from build123d import *

# Parameters (mm, degrees)
ESBO_O1_W                     = 46
ESBO_O1_H                     = 19
RESSALTO_EXTRUS_O1_DEPTH      = 1.5
CORTE_EXTRUS_O3_DEPTH         = 25.929901725
CORTE_EXTRUS_O3_DEPTH_BACK    = 25.929901725
ESBO_O6_W                     = 3
ESBO_O6_H                     = 6
CORTE_EXTRUS_O2_DEPTH         = 25.929901725
CORTE_EXTRUS_O2_DEPTH_BACK    = 25.929901725
DENTE_W                       = 3
DENTE_H                       = 3
RESSALTO_EXTRUS_O3_DEPTH      = 1.5
RESSALTO_EXTRUS_O3_DEPTH_BACK = 1.5
ESBO_O4_W                     = 3
ESBO_O4_H                     = 6
ESBO_O21_W                    = 9
ESBO_O21_H                    = 3
ESBO_O21_W_2                  = 2.5
ESBO_O21_H_2                  = 5.5
CORTE_EXTRUS_O11_DEPTH        = 3
ESBO_O3_W                     = 3
ESBO_O3_H                     = 4.5
RESSALTO_EXTRUS_O2_DEPTH      = 1.5
CORTE_EXTRUS_O12_DEPTH        = 28.721832551
CORTE_EXTRUS_O12_DEPTH_BACK   = 28.721832551
ESBO_O23_W                    = 8
ESBO_O23_H                    = 3


with BuildPart() as part:
    # Esboço1 → Ressalto-extrusão1 (new, symmetric)
    with BuildSketch(Plane.XY):
        Rectangle(ESBO_O1_W, ESBO_O1_H)
    extrude(amount=RESSALTO_EXTRUS_O1_DEPTH, both=True)

    # Esboço6 → Corte-extrusão3 (cut, two sides: drawn at the far end of the back side and taken through both)
    with BuildSketch(Plane.XY.offset(-CORTE_EXTRUS_O3_DEPTH_BACK)):
        with Locations((-3.3, -0.5)):
            Rectangle(ESBO_O6_W, ESBO_O6_H)
    extrude(amount=CORTE_EXTRUS_O3_DEPTH + CORTE_EXTRUS_O3_DEPTH_BACK, mode=Mode.SUBTRACT)

    # Dente → Corte-extrusão2 (cut, two sides: drawn at the far end of the back side and taken through both)
    with BuildSketch(Plane.XY.offset(-CORTE_EXTRUS_O2_DEPTH_BACK)):
        with Locations((5.5, -5)):
            Rectangle(DENTE_W, DENTE_H)
    extrude(amount=CORTE_EXTRUS_O2_DEPTH + CORTE_EXTRUS_O2_DEPTH_BACK, mode=Mode.SUBTRACT)

    # Esboço4 → Ressalto-extrusão3 (add, two sides: drawn at the far end of the back side and taken through both)
    with BuildSketch(Plane.XY.offset(-RESSALTO_EXTRUS_O3_DEPTH_BACK)):
        with Locations((24.5, 6.5)):
            Rectangle(ESBO_O4_W, ESBO_O4_H)
        with Locations((24.5, -6.5)):
            Rectangle(ESBO_O4_W, ESBO_O4_H)
    extrude(amount=RESSALTO_EXTRUS_O3_DEPTH + RESSALTO_EXTRUS_O3_DEPTH_BACK)

    # Esboço21 → Corte-extrusão11 (cut)
    with BuildSketch(Plane(origin=(2.822956614, -2.284701659, 1.5), x_dir=(1, 0, 0), z_dir=(0, 0, 1))):
        with Locations((-21.322956614, 2.284701659)):
            Rectangle(ESBO_O21_W, ESBO_O21_H)
        with Locations((-21.472956614, 2.284701659)):
            Rectangle(ESBO_O21_W_2, ESBO_O21_H_2)
    corte_extrus_o11 = extrude(amount=-CORTE_EXTRUS_O11_DEPTH, mode=Mode.SUBTRACT)

    # Espelhar3: Corte-extrusão11 across plane
    add(corte_extrus_o11.mirror(Plane(origin=(0, 0, 0), x_dir=(0, 0, 1), z_dir=(1, 0, 0))), mode=Mode.SUBTRACT)

    # Esboço3 → Ressalto-extrusão2 (add, symmetric)
    with BuildSketch(Plane.XY):
        with Locations((-24.5, -7.25)):
            Rectangle(ESBO_O3_W, ESBO_O3_H)
    ressalto_extrus_o2 = extrude(amount=RESSALTO_EXTRUS_O2_DEPTH, both=True)

    # Espelhar2: Corte-extrusão11, Ressalto-extrusão2 across plane
    add(corte_extrus_o11.mirror(Plane.ZX), mode=Mode.SUBTRACT)
    add(ressalto_extrus_o2.mirror(Plane.ZX))

    # Esboço23 → Corte-extrusão12 (cut, two sides: drawn at the far end of the back side and taken through both)
    with BuildSketch(Plane.XY.offset(-CORTE_EXTRUS_O12_DEPTH_BACK)):
        with Locations((7, 4)):
            Rectangle(ESBO_O23_W, ESBO_O23_H)
    extrude(amount=CORTE_EXTRUS_O12_DEPTH + CORTE_EXTRUS_O12_DEPTH_BACK, mode=Mode.SUBTRACT)


solid = part.part
Can you work these out from the model? Positions are in its coordinate system, mm. A direction names the side the tool comes from. Coordinates: 2 decimals unless noted, no trailing zeros. Write each loop counter-clockwise with the first axis right and the second up, starting at its lowest first coordinate (ties: lowest second). Pieces come first, ordered by that corner, then holes. Notation, with made-up numbers: M -6.5,-34.5 L 31.5,-34.5 A28 ccw 31.5,-8.5 Z; hole C -7,27.25 d1. An arc over 180 degrees is marked long. Use one line per item in the form item = value.
Q1. If we section it at C-C (z = -0.35): State how many separate pieces and enclosed holes the cut face has, then the cut area to 4 significant figures.
Model answer:
separate_pieces = 1
enclosed_holes = 3
area = 819.5 mm^2
Q2. I need wall thicknesses on line 1 along Y through (x, z) = (6, -1.3); line 2 along X through (y, z) = (2, -1.2); line 3 along X through (y, z) = (-3, -0.25). Which ranges of each line are inside material? Lowest first, please. Write a range as from..to.
Model answer:
line_1 = -9.5..-6.5, -3.5..2.5, 5.5..9.5
line_2 = -23..-19.9, -17.4..-4.8, -1.8..17.4, 19.9..23
line_3 = -23..-4.8, -1.8..23
Q3. If we section it at A-A (y = -2): Write out the boundary of the cut face in (x, z).
Model answer:
outline = M -23,-1.5 L -19.9,-1.5 L -19.9,1.5 L -23,1.5 Z; M -17.4,-1.5 L -4.8,-1.5 L -4.8,1.5 L -17.4,1.5 Z; M -1.8,-1.5 L 17.4,-1.5 L 17.4,1.5 L -1.8,1.5 Z; M 19.9,-1.5 L 23,-1.5 L 23,1.5 L 19.9,1.5 Z
Q4. We'd pull the mould along X, two halves only. Please class faces 4 (the flat face through (-17.4, -2, 0)), 5 (the flat face through (16, 1.5, 0)), 6 (the flat face through (23, -3, 0)): +X half, -X half, draft (parallel to the pull), parting line (faces both ways), or undercut.
Model answer:
face_4 = undercut
face_5 = draft
face_6 = +X half
Q5. For faces 1 (the flat face through (14, 0, 0)), 2 (the flat face through (-1.8, -1, 0)), 3 (the flat face through (-21, 1.5, 0)), which set-ups out of +Z, -Z, +X, -X, +Y, -Y let a thin tool reach every point of the face, with its end or its side?
Model answer:
face_1 = +Z, -Z, +X
face_2 = +Z, -Z
face_3 = +Z, -Z, -X
Q6. If we section it at B-B (x = 21.5): Write out the boundary of the cut face in (y, z), then the cut area to 3 significant figures.
Model answer:
outline = M -9.5,-1.5 L -1.5,-1.5 L -1.5,1.5 L -9.5,1.5 Z; M 1.5,-1.5 L 9.5,-1.5 L 9.5,1.5 L 1.5,1.5 Z
area = 48.0 mm^2
Q7. For P1, Ø1.4, axis at y = -2, z = 0, coming from the -X side; P2, Ø1.5, axis at y = 0.5, z = -0.5, coming from the +X side; P3, Ø1.4, axis at y = 2, z = 0.5, coming from the +X side, each with a flat end and sliding along its axis, tell me the tip position at first contact or that it passes through.
Model answer:
P1 = -23
P2 = 14
P3 = 23
